Here's how the part is built. I have some questions about the finished solid (model axes, mm). A direction names the side the tool comes from. Give positions to 0.01 mm unless a question says otherwise; leave off trailing zeros. Loops run counter-clockwise (first coordinate to the right, second up) from the corner with the lowest first, then second, coordinate; pieces in that order, holes last. Notation, with made-up numbers: (85, 77.25) - (117, 77.25) arc R13 cw to (117, 97.25) - close; hole circle Ø7 at (61, 32.25). An arc over 180 degrees is marked (long way). Use a Markdown table: item, result.
from build123d import *

# Parameters (mm, degrees)
SKETCH1_R                  = 5
BOSS_EXTRUDE1_DEPTH        = 29.5
BOSS_EXTRUDE2_DEPTH        = 3
SKETCH3_R                  = 4
CUT_EXTRUDE1_DEPTH         = 34.752777663
F_3_2_3_2_DIAMETER_HOLE1_D = 3.2


with BuildPart() as part:
    # Sketch1 → Boss-Extrude1 (new body)
    with BuildSketch(Plane(origin=(0, 0, 0), x_dir=(1, 0, 0), z_dir=(0, 1, 0))):
        with Locations(Location((0, 0, 0), (0, 0, 270))):
            Circle(SKETCH1_R)
    extrude(amount=BOSS_EXTRUDE1_DEPTH)

    # Sketch2 → Boss-Extrude2 (add)
    with BuildSketch(Plane(origin=(0, 5.5, 0), x_dir=(1, 0, 0), z_dir=(0, 1, 0))):
        with BuildLine():
            Line((8.306623863, 10), (-8.306623863, 10))
            ThreePointArc((-8.306623863, 10), (-11.768307238, 5.523309222), (-13, -2.7e-08))
            ThreePointArc((-13, -2.7e-08), (-11.768307226, -5.523309246), (-8.306623863, -10))
            Line((-8.306623863, -10), (8.306623863, -10))
            ThreePointArc((8.306623863, -10), (11.768307232, -5.523309234), (13, 0))
            ThreePointArc((13, 0), (11.768307232, 5.523309234), (8.306623863, 10))
        make_face()
    extrude(amount=BOSS_EXTRUDE2_DEPTH)

    # Sketch3 → Cut-Extrude1 (cut, through all)
    with BuildSketch(Plane(origin=(0, 29.5, 0), x_dir=(1, 0, 0), z_dir=(0, 1, 0))):
        with Locations(Location((0, 0, 0), (0, 0, 270))):
            Circle(SKETCH3_R)
    extrude(amount=-CUT_EXTRUDE1_DEPTH, mode=Mode.SUBTRACT)

    # Ø3.2 (3.2) Diameter Hole1 (through all)
    with Locations(Plane(origin=(8, 8.5, 6), x_dir=(0, 0, 1), z_dir=(0, 1, 0))):
        with Locations((0, 0), (-12, 0), (-12, -16), (0, -16)):
            Hole(F_3_2_3_2_DIAMETER_HOLE1_D / 2)


solid = part.part
(1) Suppose I cut it at A-A on x = 0. Write out the boundary of the cut face in (y, z), plus the area to 3 significant figures.
A:
| item | result |
|---|---|
| outline | (0, -5) - (5.5, -5) - (5.5, -10) - (8.5, -10) - (8.5, -5) - (29.5, -5) - (29.5, -4) - (0, -4) - close; (0, 4) - (29.5, 4) - (29.5, 5) - (8.5, 5) - (8.5, 10) - (5.5, 10) - (5.5, 5) - (0, 5) - close |
| area | 89.0 mm2 |
(2) On a 3-axis mill with a long thin cutter (end or side, diameter ignored), from which of +Z, -Z, +X, -X, +Y, -Y can I reach the whole of each face in a straight line? I mean faces 1 (the face through (-3.1, 5.5, 4.3)), 2 (the face through (6.58, 6.98, 5.26)), 3 (the face through (-4.88, 18.85, -1.08)). Say none if no direction works.
A:
| item | result |
|---|---|
| face 1 | -Y |
| face 2 | +Y, -Y |
| face 3 | +Y |
(3) Suppose I cut it at B-B on z = 2.25. Write out the boundary of the cut face in (x, y).
A:
| item | result |
|---|---|
| outline | (-12.8, 5.5) - (-4.47, 5.5) - (-4.47, 0) - (-3.31, 0) - (-3.31, 29.5) - (-4.47, 29.5) - (-4.47, 8.5) - (-12.8, 8.5) - close; (3.31, 0) - (4.47, 0) - (4.47, 5.5) - (12.8, 5.5) - (12.8, 8.5) - (4.47, 8.5) - (4.47, 29.5) - (3.31, 29.5) - close |
(4) We'd pull the mould along Z, two halves only. Please class faces 4 (the face through (-3.1, 8.5, 4.3)), 5 (the face through (-9.42, 6.98, -6.74)), 6 (the face through (0, 7, -10)), 7 (the face through (-4.88, 2.71, -1.08)): pulls with the +Z half, pulls with the -Z half, needs draft (parallel to the pull), parting line crosses it, or undercut.
A:
| item | result |
|---|---|
| face 4 | needs draft |
| face 5 | undercut |
| face 6 | pulls with the -Z half |
| face 7 | parting line crosses it |
(5) If I drill on line 1 (X direction, y = 22.25, z = 0); line 2 (X direction, y = 6.5, z = 6); line 3 (Y direction, x = -11.5, z = 5), over which ranges is the centre line in solid material (lowest first)?
A:
| item | result |
|---|---|
| line 1 | -5 to -4, 4 to 5 |
| line 2 | -11.53 to -9.6, -6.4 to 6.4, 9.6 to 11.53 |
| line 3 | 5.5 to 8.5 |
(6) Suppose I cut it at D-D on y = 14.75. Write out the boundary of the cut face in (x, z), plus the area to 3 significant figures.
A:
| item | result |
|---|---|
| outline | circle Ø10 at (0, 0); hole circle Ø8 at (0, 0) |
| area | 28.3 mm2 |
(7) Will these pins go through, and if not, where does the flat tip stop? pin 1 (2 mm diameter, centred on x = 6.5, z = -6, fed in from +Y); pin 2 (8 mm diameter, centred on x = -2.5, y = 15, fed in from +Z); pin 3 (10 mm diameter, centred on x = -8.5, y = 23.5, fed in from +Z).
A:
| item | result |
|---|---|
| pin 1 | y = 8.5 |
| pin 2 | z = 5 |
| pin 3 | z = 3.57 |
(8) Suppose I cut it at C-C on z = 6. Write out the boundary of the cut face in (x, y).
A:
| item | result |
|---|---|
| outline | (-11.53, 5.5) - (-9.6, 5.5) - (-9.6, 8.5) - (-11.53, 8.5) - close; (-6.4, 5.5) - (6.4, 5.5) - (6.4, 8.5) - (-6.4, 8.5) - close; (9.6, 5.5) - (11.53, 5.5) - (11.53, 8.5) - (9.6, 8.5) - close |
